Could you check a few things on this model? Use its own coordinates, in mm. A direction names the side the tool comes from. Round coordinates to 2 decimals unless told otherwise and drop trailing zeros. Loops run counter-clockwise (first coordinate to the right, second up) from the corner with the lowest first, then second, coordinate; pieces in that order, holes last.
from build123d import *

# Parameters (mm, degrees)
SALIENTE_EXTRUIR2_DEPTH = 2
CROQUIS3_R              = 1.5
CORTAR_EXTRUIR1_DEPTH   = 2
CROQUIS4_R              = 11
SALIENTE_EXTRUIR3_DEPTH = 3
REDONDEO1_R             = 1
REDONDEO2_R             = 1
CROQUIS6_R              = 4.927466063
CORTAR_EXTRUIR2_DEPTH   = 3
CROQUIS7_R              = 10
CORTAR_EXTRUIR3_DEPTH   = 4
REDONDEO3_R             = 3


with BuildPart() as part:
    # Croquis2 → Saliente-Extruir2 (new body)
    with BuildSketch(Plane(origin=(0, 0, 0), x_dir=(1, 0, 0), z_dir=(0, 1, 0))):
        with BuildLine():
            Line((-19, -12), (-19, -16))
            Line((-19, -16), (-15, -16))
            ThreePointArc((-15, -16), (0, -12), (15, -16))
            Line((15, -16), (19, -16))
            Line((19, -16), (19, -12))
            ThreePointArc((19, -12), (15, 0), (19, 12))
            Line((19, 12), (19, 16))
            Line((19, 16), (15, 16))
            ThreePointArc((15, 16), (0, 12), (-15, 16))
            Line((-15, 16), (-19, 16))
            Line((-19, 16), (-19, 12))
            ThreePointArc((-19, 12), (-15, 0), (-19, -12))
        make_face()
    extrude(amount=SALIENTE_EXTRUIR2_DEPTH)

    # Croquis3 → Cortar-Extruir1 (cut)
    with BuildSketch(Plane(origin=(0, 2, 0), x_dir=(1, 0, 0), z_dir=(0, 1, 0))):
        with Locations(Location((-17, 14, 0), (0, 0, 270))):
            Circle(CROQUIS3_R)
        with Locations(Location((17, 14, 0), (0, 0, 270))):
            Circle(CROQUIS3_R)
        with Locations(Location((17, -14, 0), (0, 0, 270))):
            Circle(CROQUIS3_R)
        with Locations(Location((-17, -14, 0), (0, 0, 270))):
            Circle(CROQUIS3_R)
    extrude(amount=-CORTAR_EXTRUIR1_DEPTH, mode=Mode.SUBTRACT)

    # Croquis4 → Saliente-Extruir3 (add)
    with BuildSketch(Plane(origin=(0, 2, 0), x_dir=(1, 0, 0), z_dir=(0, 1, 0))):
        with Locations(Location((0, 0, 0), (0, 0, 90))):
            Circle(CROQUIS4_R)
    extrude(amount=SALIENTE_EXTRUIR3_DEPTH)

    # Redondeo1
    redondeo1_edges = [part.edges().sort_by_distance(p)[0] for p in [
        (0, 5, 11),
    ]]
    fillet(redondeo1_edges, radius=REDONDEO1_R)

    # Redondeo2
    redondeo2_edges = [part.edges().sort_by_distance(p)[0] for p in [
        (0, 2, 11),
    ]]
    fillet(redondeo2_edges, radius=REDONDEO2_R - 0.0001)  # a hair under: the kernel refuses the full size

    # Croquis6 → Cortar-Extruir2 (cut)
    with BuildSketch(Plane(origin=(0, 5, 0), x_dir=(1, 0, 0), z_dir=(0, 1, 0))):
        with Locations(Location((0, 0, 0), (0, 0, 270))):
            Circle(CROQUIS6_R)
    extrude(amount=-CORTAR_EXTRUIR2_DEPTH, mode=Mode.SUBTRACT)

    # Croquis7 → Cortar-Extruir3 (cut)
    with BuildSketch(Plane.XZ):
        with Locations(Location((0, 0, 0), (0, 0, 270))):
            Circle(CROQUIS7_R)
    extrude(amount=-CORTAR_EXTRUIR3_DEPTH, mode=Mode.SUBTRACT)

    # Redondeo3
    redondeo3_edges = [part.edges().sort_by_distance(p)[0] for p in [
        (0, 4, 10),
    ]]
    fillet(redondeo3_edges, radius=REDONDEO3_R)


solid = part.part
Item 1: Will these pins go through, and if not, where does the flat tip stop? pin 1 (11 mm diameter, centred on x = -0.5, z = 1.5, fed in from -Y); pin 2 (4 mm diameter, centred on x = -17, z = -14, fed in from -Y); pin 3 (2.5 mm diameter, centred on x = -17, z = 14, fed in from -Y); pin 4 (18 mm diameter, centred on x = 0, z = 0, fed in from -Y).
Results list:
pin 1: stops at y = 4
pin 2: stops at y = 0
pin 3: passes through
pin 4: stops at y = 3.24
Item 2: For faces 4 (the cylindrical face through (10.74, 3.49, 2.38)), 5 (the flat face through (-17, 1, 16)), which set-ups out of +Z, -Z, +X, -X, +Y, -Y let a thin tool reach every point of the face, with its end or its side?
Results list:
face 4: +Y
face 5: +Z, +X, -X, +Y, -Y
Item 3: If we section it at D-D, the plane z = -14: Please give me the cut outline in (x, y), then the cut area to 3 significant figures.
Results list:
outline: (-19, 0) - (-18.5, 0) - (-18.5, 2) - (-19, 2) - close; (-15.5, 0) - (-10.79, 0) - (-10.79, 2) - (-15.5, 2) - close; (10.79, 0) - (15.5, 0) - (15.5, 2) - (10.79, 2) - close; (18.5, 0) - (19, 0) - (19, 2) - (18.5, 2) - close
area: 20.8 mm2
Item 4: If we section it at B-B, the plane x = 16.5: Please give me the cut outline in (y, z).
Results list:
outline: (0, -16) - (2, -16) - (2, -15.41) - (0, -15.41) - close; (0, -12.59) - (2, -12.59) - (2, -7.6) - (0, -7.6) - close; (0, 7.6) - (2, 7.6) - (2, 12.59) - (0, 12.59) - close; (0, 15.41) - (2, 15.41) - (2, 16) - (0, 16) - close
Item 5: If I drill on line 1 along Y through (x, z) = (11, 6); line 2 along Z through (x, y) = (6, 0.9); line 3 along X through (y, z) = (4.05, 4.5), over which ranges is the centre line in solid material (lowest first)?
Results list:
line 1: y = 0 to 2
line 2: z = -12.6 to -8, 8 to 12.6
line 3: x = -10.04 to -2.01, 2.01 to 10.04
Item 6: If we section it at A-A, the plane z = 0: Please give me the cut outline in (x, y), then the cut area to 3 significant figures.
Results list:
outline: (-15, 0) - (-10, 0) - (-10, 1) arc R3 cw to (-7, 4) - (-4.93, 4) - (-4.93, 5) - (-10, 5) arc R1 ccw to (-11, 4) - (-11, 3) arc R1 cw to (-12, 2) - (-15, 2) - close; (4.93, 4) - (7, 4) arc R3 cw to (10, 1) - (10, 0) - (15, 0) - (15, 2) - (12, 2) arc R1 cw to (11, 3) - (11, 4) arc R1 ccw to (10, 5) - (4.93, 5) - close
area: 40.0 mm2
Item 7: We'd pull the mould along Z, two halves only. Please class faces 1 (the cylindrical face through (0, 1, 12)), 2 (the flat face through (-17, 1, -16)), 3 (the cylindrical face through (1.48, 4.51, 4.7)): released by +Z, released by -Z, zero draft, split by the parting line, or undercut.
Results list:
face 1: released by +Z
face 2: released by -Z
face 3: undercut
